Build history of the part. All positions in model axes, mm. A direction names the side the tool comes from. Give positions to 0.01 mm unless a question says otherwise; leave off trailing zeros. Order: outer loops, then holes, each group sorted by start corner. A loop starts at its lowest first (then second) coordinate and runs counter-clockwise, first axis right, second up. Notation, with made-up numbers: (39, -10) - (44, -10) arc R22 cw to (44, 29) - close; hole circle Ø6 at (46, 59.25). An arc over 180 degrees is marked (long way). One line per item, written item: value.
```python
from build123d import *

# Parameters (mm, degrees)
F1_DEPTH = 40.2336
F0_R     = 10.16
F2_DEPTH = 15.7734
F3_R     = 3.302


with BuildPart() as f1:
    # F0 (on Top) → F1 (new body)
    with BuildSketch(Plane.XY):
        with BuildLine():
            ThreePointArc((-38.632684, -28.118692), (-21.788691, -18.319272), (-15.143919, 0))
            ThreePointArc((-15.143919, 0), (-21.788691, 18.319272), (-38.632684, 28.118692))
            ThreePointArc((-38.632684, 28.118692), (-72.293919, 0), (-38.632684, -28.118692))
        make_face()
        with BuildLine():
            ThreePointArc((-30.439394, -5.271326), (-58.006419, 0), (-30.439394, 5.271326))
            Line((-30.439394, 5.271326), (-24.181643, 5.271326))
            Line((-24.181643, 5.271326), (-24.181643, -5.271326))
            Line((-24.181643, -5.271326), (-30.439394, -5.271326))
        make_face(mode=Mode.SUBTRACT)
    extrude(amount=F1_DEPTH)

    # F0 (on Top) → F2 (join)
    with BuildSketch(Plane.XY):
        with BuildLine():
            ThreePointArc((-38.632684, -28.118692), (-21.788691, -18.319272), (-15.143919, 0))
            ThreePointArc((-15.143919, 0), (-21.788691, 18.319272), (-38.632684, 28.118692))
            ThreePointArc((-38.632684, 28.118692), (-72.293919, 0), (-38.632684, -28.118692))
        make_face()
        with BuildLine():
            ThreePointArc((-30.439394, -5.271326), (-58.006419, 0), (-30.439394, 5.271326))
            Line((-30.439394, 5.271326), (-24.181643, 5.271326))
            Line((-24.181643, 5.271326), (-24.181643, -5.271326))
            Line((-24.181643, -5.271326), (-30.439394, -5.271326))
        make_face(mode=Mode.SUBTRACT)
        with BuildLine():
            ThreePointArc((-38.632684, 28.118692), (-21.788691, 18.319272), (-15.143919, 0))
            ThreePointArc((-15.143919, 0), (-21.788691, -18.319272), (-38.632684, -28.118692))
            Line((-38.632684, -28.118692), (11.891298, -18.979688))
            ThreePointArc((11.891298, -18.979688), (29.306081, 0), (11.891298, 18.979688))
            Line((11.891298, 18.979688), (-38.632684, 28.118692))
        make_face()
        with Locations((10.256081, 0)):
            Circle(F0_R, mode=Mode.SUBTRACT)
    extrude(amount=F2_DEPTH)

    # F3
    f3_edges = [f1.edges().sort_by_distance(p)[0] for p in [
        (-48.805153, 28.118692, 40.2336),
    ]]
    fillet(f3_edges, radius=F3_R)


solid = f1.part
```
(1) Drill centre lines: line 1 (Z direction, x = -67, y = 10.5); line 2 (Y direction, x = -56.5, z = 19); line 3 (Y direction, x = -54, z = 35). Where is each one in solid material? Low to high.
Completed:
line 1: 0 to 40.22
line 2: -25.56 to -6.39, 6.39 to 25.56
line 3: -26.66 to -9.92, 9.92 to 26.66
(2) 3-axis set-ups, long thin cutter, end or side, ignore diameter. For faces 4 (the face through (-33, -11, 40.234)), 5 (the face through (-24.182, 0, 20)): which of +Z, -Z, +X, -X, +Y, -Y reach the whole face in a straight line?
Completed:
face 4: +Z, +X, -X, +Y, -Y
face 5: +Z, -Z
(3) Slice it at B-B, the plane x = 10. Give the cut face in (y, z), and give its area (3 significant figures).
Completed:
outline: (-19.32, 0) - (-10.16, 0) - (-10.16, 15.77) - (-19.32, 15.77) - close; (10.16, 0) - (19.32, 0) - (19.32, 15.77) - (10.16, 15.77) - close
area: 289 mm²
(4) Slice it at C-C, the plane y = -2.5. Count the separate pieces of the cut face and the enclosed holes in it, and give its area (3 significant figures).
Completed:
separate pieces: 3
enclosed holes: 0
area: 1,320 mm²
(5) Pull direction X, two halves, no side cores. Call faces 1 (the face through (-22, 0, 0)), 2 (the face through (-13.017, 23.485, 7.776)), 3 (the face through (-27, -5.271, 20)): +X half, -X half, draft (parallel to the pull), parting line (faces both ways), or undercut.
Completed:
face 1: draft
face 2: +X half
face 3: undercut
(6) Pin check, flat tips, straight feed: P1, Ø17, axis at x = -8.5, y = 7.5, coming from the +Z side; P2, Ø5.5, axis at y = -2.5, z = 26, coming from the -X side; P3, Ø3, axis at x = -28.5, z = 20.5, coming from the +Y side; P4, Ø18.5, axis at x = 10.26, y = 0, coming from the +Z side. Stop position of each tip, or through.
Completed:
P1: z = 39.36
P2: x = -72.29
P3: y = 25.07
P4: through
